from build123d import *

# Parameters (mm, degrees)
CROQUIS1_W              = 90
CROQUIS1_H              = 80
SALIENTE_EXTRUIR1_DEPTH = 50
CROQUIS2_W              = 85
CROQUIS2_H              = 80
CORTAR_EXTRUIR1_DEPTH   = 23
CROQUIS3_W              = 61.032840672
CROQUIS3_H              = 80
CORTAR_EXTRUIR2_DEPTH   = 32
CROQUIS4_W              = 23.967159328
CROQUIS4_H              = 70
CORTAR_EXTRUIR3_DEPTH   = 22
CROQUIS7_R              = 6.77
CORTAR_EXTRUIR6_DEPTH   = 10
CROQUIS11_W             = 13
CROQUIS11_H             = 70
SALIENTE_EXTRUIR2_DEPTH = 2
CROQUIS12_W             = 13
CROQUIS12_H             = 55
SALIENTE_EXTRUIR3_DEPTH = 5
REDONDEO3_R             = 12
REDONDEO4_R             = 12
CROQUIS14_W             = 13
CROQUIS14_H             = 13
SALIENTE_EXTRUIR4_DEPTH = 1
CROQUIS17_W             = 2.726828244
CROQUIS17_H             = 50
SALIENTE_EXTRUIR5_DEPTH = 1.6
CROQUIS18_W             = 5
CROQUIS18_H             = 50
SALIENTE_EXTRUIR6_DEPTH = 1
CHAFL_N2_SIZE           = 4
CHAFL_N4_SIZE           = 4
CROQUIS19_R             = 2.165
CORTAR_EXTRUIR10_DEPTH  = 10
CROQUIS20_W             = 5.4
CROQUIS20_H             = 1.857846889
CORTAR_EXTRUIR11_DEPTH  = 80
REDONDEO10_R            = 10
CROQUIS23_W             = 40.8
CROQUIS23_H             = 20.5
CORTAR_EXTRUIR12_DEPTH  = 22
CROQUIS24_W             = 5
CROQUIS24_H             = 80
CORTAR_EXTRUIR14_DEPTH  = 2
REDONDEO13_R            = 16
REDONDEO14_START        = 30
REDONDEO14_DEPTH        = 2.2192
REDONDEO14_START_2      = 32.2192
REDONDEO14_2_DEPTH      = 7.7808
REDONDEO14_START_3      = -40
REDONDEO14_3_DEPTH      = 14.749021125
CORTAR_EXTRUIR16_DEPTH  = 1.3
CHAFL_N5_SIZE           = 5


with BuildPart() as part:
    # Croquis1 → Saliente-Extruir1 (new body)
    with BuildSketch(Plane(origin=(0, 0, 0), x_dir=(1, 0, 0), z_dir=(0, 1, 0))):
        Rectangle(CROQUIS1_W, CROQUIS1_H)
    extrude(amount=SALIENTE_EXTRUIR1_DEPTH)

    # Croquis2 → Cortar-Extruir1 (cut)
    with BuildSketch(Plane(origin=(0, 50, 0), x_dir=(1, 0, 0), z_dir=(0, 1, 0))):
        with Locations((2.5, 0)):
            Rectangle(CROQUIS2_W, CROQUIS2_H)
    extrude(amount=-CORTAR_EXTRUIR1_DEPTH, mode=Mode.SUBTRACT)

    # Croquis3 → Cortar-Extruir2 (cut)
    with BuildSketch(Plane(origin=(0, 27, 0), x_dir=(1, 0, 0), z_dir=(0, 1, 0))):
        with Locations((14.483579664, 0)):
            Rectangle(CROQUIS3_W, CROQUIS3_H)
    extrude(amount=-CORTAR_EXTRUIR2_DEPTH, mode=Mode.SUBTRACT)

    # Croquis4 → Cortar-Extruir3 (cut)
    with BuildSketch(Plane(origin=(0, 27, 0), x_dir=(1, 0, 0), z_dir=(0, 1, 0))):
        with Locations((-28.016420336, 5)):
            Rectangle(CROQUIS4_W, CROQUIS4_H)
    extrude(amount=-CORTAR_EXTRUIR3_DEPTH, mode=Mode.SUBTRACT)

    # Croquis7 → Cortar-Extruir6 (cut)
    with BuildSketch(Plane.XY.offset(40)):
        with Locations((-28.569213332, 14.444335644)):
            Circle(CROQUIS7_R)
    extrude(amount=-CORTAR_EXTRUIR6_DEPTH, mode=Mode.SUBTRACT)

    # Croquis11 → Saliente-Extruir2 (add)
    with BuildSketch(Plane(origin=(0, 5, 0), x_dir=(1, 0, 0), z_dir=(0, 1, 0))):
        with Locations((-28.016420336, 5)):
            Rectangle(CROQUIS11_W, CROQUIS11_H)
    extrude(amount=SALIENTE_EXTRUIR2_DEPTH)

    # Croquis12 → Saliente-Extruir3 (add)
    with BuildSketch(Plane(origin=(0, 7, 0), x_dir=(1, 0, 0), z_dir=(0, 1, 0))):
        with Locations((-28.016420336, 12.5)):
            Rectangle(CROQUIS12_W, CROQUIS12_H)
    extrude(amount=SALIENTE_EXTRUIR3_DEPTH)

    # Redondeo3
    # the kernel refuses this fillet: 12 mm, written as the material it adds along each edge
    with BuildSketch(Plane(origin=(-40, 5, 30), x_dir=(1.0, 1.01847082473682e-12, 0), z_dir=(0, 0, -1))) as redondeo3_piece_1:
        with BuildLine():
            CenterArc((12, -10.076520531), REDONDEO3_R, 122.890486336, 57.109513664)
            Line((0, -10.076520531), (-0.24, -10.076520531))
            Line((-0.24, -10.076520531), (-0.24, 0))
            Line((-0.24, 0), (0, 0.24))
            ThreePointArc((0, 0.24), (2.741789832, 0.24), (5.353251257, 0.201530411))
            Line((5.353251257, 0.201530411), (5.483579664, 0))
        make_face()
    extrude(amount=70)

    # Redondeo4
    redondeo4_edges = [part.edges().sort_by_distance(p)[0] for p in [
        (-45, 0, 0),
    ]]
    fillet(redondeo4_edges, radius=REDONDEO4_R)

    # Croquis14 → Saliente-Extruir4 (add)
    with BuildSketch(Plane(origin=(0, 7, 0), x_dir=(1, 0, 0), z_dir=(0, 1, 0))):
        with Locations((-28.016420336, -21.5)):
            Rectangle(CROQUIS14_W, CROQUIS14_H)
    extrude(amount=SALIENTE_EXTRUIR4_DEPTH)

    # Croquis17 → Saliente-Extruir5 (add)
    with BuildSketch(Plane(origin=(0, 12, 0), x_dir=(1, 0, 0), z_dir=(0, 1, 0))):
        with Locations((-22.879834458, 15)):
            Rectangle(CROQUIS17_W, CROQUIS17_H)
    extrude(amount=SALIENTE_EXTRUIR5_DEPTH)

    # Croquis18 → Saliente-Extruir6 (add)
    with BuildSketch(Plane(origin=(0, 13.6, 0), x_dir=(1, 0, 0), z_dir=(0, 1, 0))):
        with Locations((-24.016420336, 15)):
            Rectangle(CROQUIS18_W, CROQUIS18_H)
    extrude(amount=SALIENTE_EXTRUIR6_DEPTH)

    # Chaflán2
    chafl_n2_edges = [part.edges().sort_by_distance(p)[0] for p in [
        (-28.016420336, 12, 15),
    ]]
    chamfer(chafl_n2_edges, length=CHAFL_N2_SIZE - 0.0001)  # a hair under: the kernel refuses the full size

    # Chaflán4
    chafl_n4_edges = [part.edges().sort_by_distance(p)[0] for p in [
        (-24.016420336, 14.6, -40),
    ]]
    chamfer(chafl_n4_edges, length=CHAFL_N4_SIZE)

    # Croquis19 → Cortar-Extruir10 (cut)
    with BuildSketch(Plane.ZY.offset(45)):
        with Locations((-24.340228639, 34.810686035)):
            Circle(CROQUIS19_R)
        with Locations((-24.340228639, 24.860686035)):
            Circle(CROQUIS19_R)
        with Locations((22.759771361, 34.810686035)):
            Circle(CROQUIS19_R)
        with Locations((22.759771361, 24.860686035)):
            Circle(CROQUIS19_R)
    extrude(amount=-CORTAR_EXTRUIR10_DEPTH, mode=Mode.SUBTRACT)

    # Croquis20 → Cortar-Extruir11 (cut)
    with BuildSketch(Plane(origin=(0, 0, -40), x_dir=(-1, 0, 0), z_dir=(0, 0, -1))):
        with Locations((28.569213332, 11.071076555)):
            Rectangle(CROQUIS20_W, CROQUIS20_H)
    extrude(amount=-CORTAR_EXTRUIR11_DEPTH, mode=Mode.SUBTRACT)

    # Redondeo10
    redondeo10_edges = [part.edges().sort_by_distance(p)[0] for p in [
        (-16.032840672, 27, 35),
    ]]
    fillet(redondeo10_edges, radius=REDONDEO10_R)

    # Croquis23 → Cortar-Extruir12 (cut)
    with BuildSketch(Plane(origin=(-40, 0, 0), x_dir=(0, 0, -1), z_dir=(1, 0, 0))):
        with Locations((0.790228639, 29.835686035)):
            Rectangle(CROQUIS23_W, CROQUIS23_H)
    extrude(amount=-CORTAR_EXTRUIR12_DEPTH, mode=Mode.SUBTRACT)

    # Croquis24 → Cortar-Extruir14 (cut)
    with BuildSketch(Plane(origin=(0, 50, 0), x_dir=(1, 0, 0), z_dir=(0, 1, 0))):
        with Locations((-42.5, 0)):
            Rectangle(CROQUIS24_W, CROQUIS24_H)
    extrude(amount=-CORTAR_EXTRUIR14_DEPTH, mode=Mode.SUBTRACT)

    # Redondeo13
    redondeo13_edges = [part.edges().sort_by_distance(p)[0] for p in [
        (-42.5, 48, -40),
        (-42.5, 48, 40),
    ]]
    fillet(redondeo13_edges, radius=REDONDEO13_R)

    # Redondeo14: read off the stored shape, not the designer's step
    # Redondeo14 outline → Redondeo14 (add)
    with BuildSketch(Plane.XY.offset(REDONDEO14_START)):
        with BuildLine():
            ThreePointArc((-26.032840672, 27), (-25.641610248, 26.992344007), (-25.250978875, 26.969387751))
            ThreePointArc((-25.250978875, 26.969387751), (-35.747673429, 32.057988118), (-40, 42.920408153))
            Line((-40, 42.920408153), (-40, 27))
            Line((-40, 27), (-26.032840672, 27))
        make_face()
    extrude(amount=REDONDEO14_DEPTH)

    # Redondeo14 2 outline → Redondeo14 2 (add)
    with BuildSketch(Plane.XY.offset(REDONDEO14_START_2)):
        with BuildLine():
            ThreePointArc((-26.032840672, 27), (-25.641610248, 26.992344007), (-25.250978875, 26.969387751))
            ThreePointArc((-25.250978875, 26.969387751), (-35.747673429, 32.057988118), (-40, 42.920408153))
            Line((-40, 42.920408153), (-40, 27))
            Line((-40, 27), (-26.032840672, 27))
        make_face()
    extrude(amount=REDONDEO14_2_DEPTH)

    # Redondeo14 3 outline → Redondeo14 3 (cut)
    with BuildSketch(Plane.YZ.offset(REDONDEO14_START_3)):
        with BuildLine():
            Line((31, 40), (32, 40))
            ThreePointArc((32, 40), (38.583005244, 38.583005244), (44, 34.583005244))
            Line((44, 34.583005244), (44, 41))
            Line((44, 41), (31, 41))
            Line((31, 41), (31, 40))
        make_face()
    extrude(amount=REDONDEO14_3_DEPTH, mode=Mode.SUBTRACT)

    # Croquis25 → Cortar-Extruir16 (cut)
    with BuildSketch(Plane.ZY.offset(26.516420336)):
        Polygon((-36, 14.6), (10, 14.6), (10, 13.6), (-37, 13.6), align=None)
    extrude(amount=-CORTAR_EXTRUIR16_DEPTH, mode=Mode.SUBTRACT)

    # Chaflán5
    # the kernel refuses this chamfer: 5 mm, written as the material it takes off along each edge
    with BuildSketch(Plane(origin=(-8.658005396, 14.6, 10), x_dir=(0, 0, -1), z_dir=(-1, 0, 0))) as chafl_n5_piece_1_section:
        Polygon((CHAFL_N5_SIZE, 0), (0, CHAFL_N5_SIZE), (0, 0), align=None)
    chafl_n5_piece_1 = extrude(amount=29.41682988, mode=Mode.PRIVATE)
    chafl_n5_piece_1 = split(chafl_n5_piece_1, bisect_by=Plane(origin=(-8.658005396, 12, 10), z_dir=(0, 1, 0)), keep=Keep.TOP, mode=Mode.PRIVATE)
    add(chafl_n5_piece_1, mode=Mode.SUBTRACT)


solid = part.part
Geometry: final body of the model. Coordinates: model frame, mm. A direction names the side the tool comes from. Give positions to 0.01 mm unless a question says otherwise; leave off trailing zeros. Loops run counter-clockwise (first coordinate to the right, second up) from the corner with the lowest first, then second, coordinate; pieces in that order, holes last. Notation, with made-up numbers: (9, 47.5) - (30, 47.5) arc R19 ccw to (30, 54.5) - close; hole circle Ø2 at (48.5, 0). An arc over 180 degrees is marked (long way). One line per question, with ' | ' between items. Start each with the question number.
(1) Pull-direction query (Z, two-part tool) for faces 6 (the flat face through (-42, 40.086, -1)), 7 (the cylindrical face through (-42.465, 43.437, -35.189)), 8 (the cylindrical face through (-22.112, 16.478, 35.07)), 9 (the flat face through (-28, 10, 13)); classes: released by +Z, released by -Z, zero draft, split by the parting line, or undercut.
(2) Section query B-B on z = -34. Return loops of the section in (x, y).
(3) Ray query, line 1 (X direction, y = 14.5, z = -21.5); line 2 (Y direction, x = -42.75, z = -1.5); line 3 (Y direction, x = -24.5, z = 0). Return the intervals inside material, ascending. Write a range as from..to.
(4) Section query C-C on x = -41.25. Return loops of the section in (y, z) (3 decimals), then the cut area to 3 significant figures.
(5) Contact query for flat-ended pins moving along their axis: pin 1 (1.5 mm diameter, centred on y = 25, z = 24, fed in from -X); pin 2 (2 mm diameter, centred on x = -23, z = -13, fed in from +Y); pin 3 (1.6 mm diameter, centred on x = -18, z = -15, fed in from +Y); pin 4 (3.5 mm diameter, centred on y = 7.5, z = -11, fed in from -X). Output: stop coordinate, or through.
(6) Section query D-D on z = 32. Return loops of the section in (x, y).
(7) Reachability of faces 1 (the flat face through (-40, 43, -10)), 2 (the flat face through (-24.243, 13, -15)), 3 (the flat face through (-28, 8, 21)), 4 (the cylindrical face through (-18.62, 23.71, 34.93)), 5 (the flat face through (-42, 30, 19.61)) from +Z, -Z, +X, -X, +Y, -Y: full face, straight path, thin tool, end or side. Return the list, or none.
(8) Section query A-A on z = -15.5. Return loops of the section in (x, y).
The answers:
1) face 6: undercut | face 7: released by -Z | face 8: zero draft | face 9: undercut
2) outline: (-45, 12) arc R12 ccw to (-33, 0) - (-16.03, 0) - (-16.03, 5) - (-21.52, 5) - (-21.52, 14.6) - (-25.22, 14.6) - (-25.22, 13.6) - (-24.24, 13.6) - (-24.24, 12) - (-25.87, 12) - (-25.87, 10.14) - (-31.27, 10.14) - (-31.27, 12) - (-34.52, 12) - (-34.52, 5) arc R12 cw to (-40, 15.08) - (-40, 44.49) - (-45, 44.49) - close
3) line 1: -45..-39.99, -25.22..-21.52 | line 2: 5..19.59, 40.09..48 | line 3: 0..12, 13.6..14.6
4) outline: (3.286, -40) - (32, -40) arc R16 ccw to (48, -24) - (48, 24) arc R16 ccw to (32, 40) - (3.286, 40) - close; hole (19.586, -21.19) - (40.086, -21.19) - (40.086, 19.61) - (19.586, 19.61) - close; hole circle Ø4.33 at (24.861, -24.34); hole circle Ø4.33 at (24.861, 22.76); hole circle Ø4.33 at (34.811, -24.34); hole circle Ø4.33 at (34.811, 22.76) | area: 2,570 mm2
5) pin 1: through | pin 2: y = 14.6 | pin 3: y = 5 | pin 4: x = -44.68
6) outline: (-45, 12) arc R12 ccw to (-33, 0) - (-16.03, 0) - (-16.03, 17) arc R10 ccw to (-25.25, 26.97) arc R16 cw to (-40, 42.92) - (-40, 45.86) - (-45, 45.86) - close; hole circle Ø13.54 at (-28.57, 14.44)
7) face 1: -Z, +X, +Y | face 2: +Z, -Z | face 3: +X, +Y | face 4: +Z, -Z, +X, +Y | face 5: +X, -X
8) outline: (-45, 12) arc R12 ccw to (-33, 0) - (-16.03, 0) - (-16.03, 5) - (-21.52, 5) - (-21.52, 14.6) - (-25.22, 14.6) - (-25.22, 13.6) - (-24.24, 13.6) - (-24.24, 12) - (-25.87, 12) - (-25.87, 10.14) - (-31.27, 10.14) - (-31.27, 12) - (-34.52, 12) - (-34.52, 5) arc R12 cw to (-40, 15.08) - (-40, 19.59) - (-45, 19.59) - close; (-45, 40.09) - (-40, 40.09) - (-40, 48) - (-45, 48) - close
